Verification items for this drawing (mm, ordinates from the low corner). Coordinates: 2 decimals unless noted, no trailing zeros. Loops run counter-clockwise (first coordinate to the right, second up) from the corner with the lowest first, then second, coordinate; pieces in that order, holes last. Notation, with made-up numbers: M 43.5,81 L 102.5,81 A26 ccw 102.5,102 Z; hole C 53.25,33.5 d10. An arc over 180 degrees is marked long. Write each question's results on one line, items separated by ' | '. Start each with the question number.
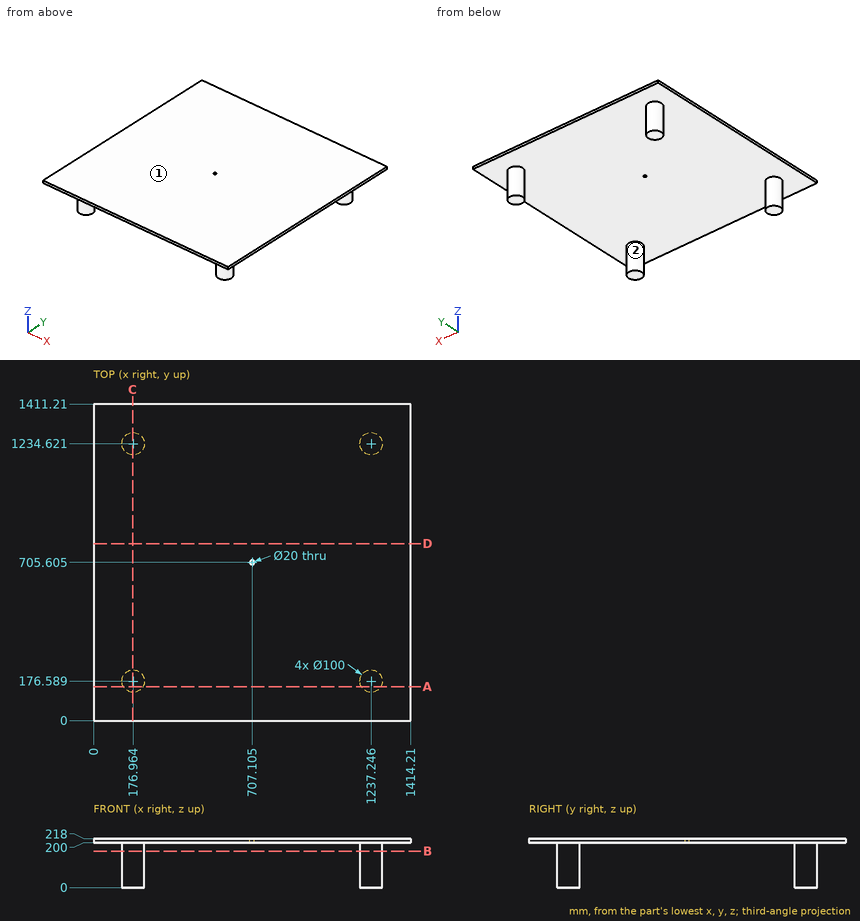
Item 1: Section check A-A (y = 152). Record the cut outline in (x, z), plus the area to 3 significant figures.
Item 2: Depth check by flat-ended pin: P1, Ø5, axis at x = 1225.5, y = 194, coming from the -Z side; P2, Ø2, axis at y = 1228.5, z = 165.5, coming from the +X side; P3, Ø3, axis at x = 1204, z = 77.5, coming from the +Y side. Enter the tip coordinate at first touch or a pass-through.
Item 3: Thickness scan on line 1 (Z direction, x = 1129, y = 1158.5); line 2 (X direction, y = 1220, z = 177); line 3 (Y direction, x = 188, z = 166) (1 decimal). Record the ranges inside material, lowest first.
Item 4: Section check D-D (y = 789). Record the cut outline in (x, z).
Item 5: Section check B-B (z = 162). Record the cut outline in (x, y), plus the area to 3 significant figures.
Item 6: Release check for a two-part mould opening along X. For the marked faces 1 and 2 record: +X half, -X half, draft (parallel to the pull), parting line (faces both ways), or undercut.
Item 7: Section check C-C (x = 174). Record the cut outline in (y, z).
Computed values:
1) outline: M 0,200 L 133.43,200 L 133.43,0 L 220.5,0 L 220.5,200 L 1193.71,200 L 1193.71,0 L 1280.78,0 L 1280.78,200 L 1414.21,200 L 1414.21,218 L 0,218 Z | area: 60,300 mm²
2) P1: stops at z = 0 | P2: stops at x = 1286.98 | P3: stops at y = 1273.25
3) line 1: z = 200 to 218 | line 2: x = 129.15 to 224.78, 1189.43 to 1285.06 | line 3: y = 127.8 to 225.4, 1185.9 to 1283.4
4) outline: M 0,200 L 1414.21,200 L 1414.21,218 L 0,218 Z
5) outline: C 176.96,176.59 d100; C 176.96,1234.62 d100; C 1237.25,176.59 d100; C 1237.25,1234.62 d100 | area: 31,400 mm²
6) face 1: draft | face 2: undercut
7) outline: M 0,200 L 126.68,200 L 126.68,0 L 226.5,0 L 226.5,200 L 1184.71,200 L 1184.71,0 L 1284.53,0 L 1284.53,200 L 1411.21,200 L 1411.21,218 L 0,218 Z
